Geometry check sheet. Reference: drawing and pictorial views, mm from the part's lowest x, y, z. A direction names the side the tool comes from. Round coordinates to 2 decimals unless told otherwise and drop trailing zeros. Write each loop counter-clockwise with the first axis right and the second up, starting at its lowest first coordinate (ties: lowest second). Pieces come first, ordered by that corner, then holes. Notation, with made-up numbers: (33.25, -37.75) - (63.25, -37.75) arc R8 ccw to (63.25, -31.75) - close; hole circle Ø1 at (65.25, -30). An arc over 180 degrees is marked (long way). Use one line per item in the form item = value. Start each with the question number.
1) Set-up check for the marked faces 4, 5 and 6: record each of +Z, -Z, +X, -X, +Y, -Y from which the full face is reachable in a straight line by a thin tool's end or side.
2) Section check B-B (y = 16). Record the boundary of the cut face in (x, z), then the cut area to 3 significant figures.
3) Section check C-C (x = 51). Record the boundary of the cut face in (y, z), then the cut area to 3 significant figures.
4) Gauge pin test, flat ends, axial feed: P1, Ø4, axis at x = 24, z = 19.5, coming from the +Y side; P2, Ø3, axis at y = 35, z = 13.5, coming from the +X side; P3, Ø12, axis at y = 13, z = 4, coming from the -X side; P4, Ø16, axis at y = 61, z = 14.5, coming from the +X side. Record the tip position at first contact, or that the pin passes through.
5) Draft check along X on the marked faces 1, 2 and 3. Enter one of: +X half, -X half, draft (parallel to the pull), parting line (faces both ways), or undercut.
6) Section check A-A (z = 7.75). Record the boundary of the cut face in (x, y).
7) Scan lines: probe 1 along Y at (x, z) = (48, 9.25); probe 2 along Z at (x, y) = (8.5, 44.5); probe 3 along Y at (x, z) = (6, 21.25). Record each from-to range of solid material in increasing order.
8) Section check D-D (x = 4). Record the boundary of the cut face in (y, z), then the cut area to 3 significant figures.
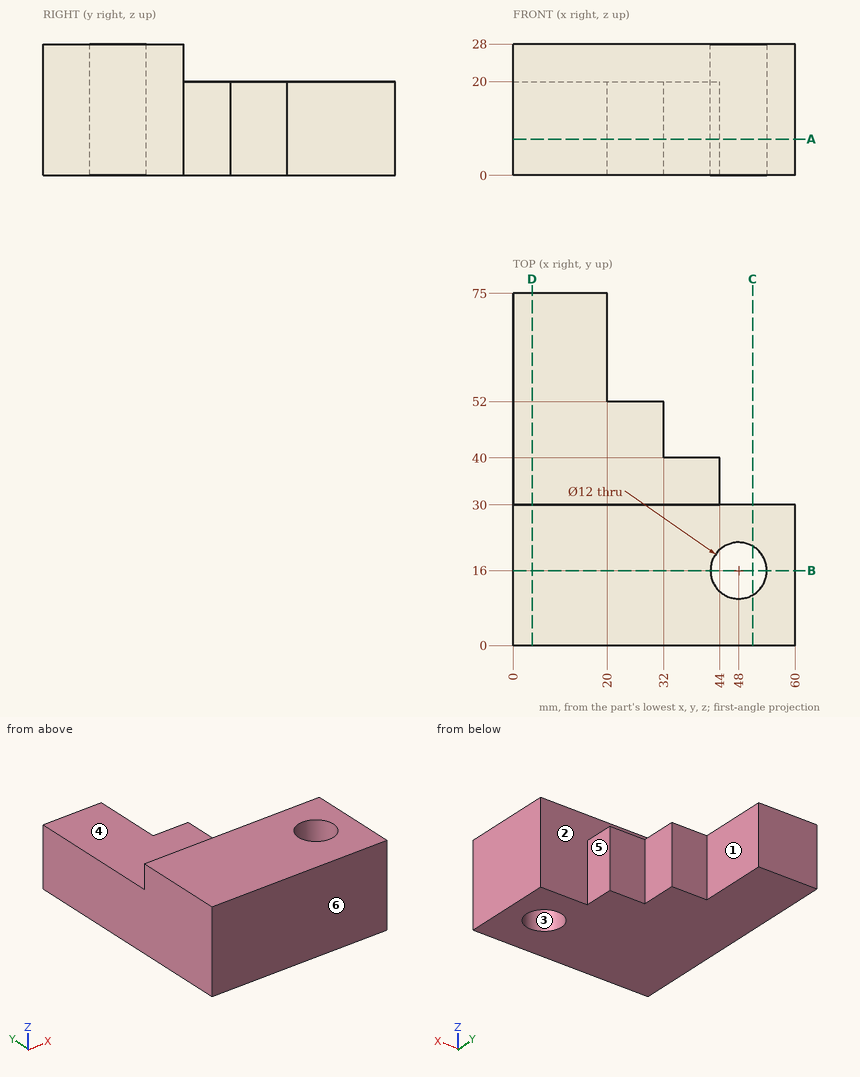
Results are:
q1.face_4 = +Z, +X, -X, +Y
q1.face_5 = +Z, -Z, +X, +Y
q1.face_6 = +Z, -Z, +X, -X, -Y
q2.outline = (0, 0) - (42, 0) - (42, 28) - (0, 28) - close; (54, 0) - (60, 0) - (60, 28) - (54, 28) - close
q2.area = 1,340 mm²
q3.outline = (0, 0) - (10.8, 0) - (10.8, 28) - (0, 28) - close; (21.2, 0) - (30, 0) - (30, 28) - (21.2, 28) - close
q3.area = 549 mm²
q4.P1 = 52
q4.P2 = 44
q4.P3 = 0
q4.P4 = 20
q5.face_1 = +X half
q5.face_2 = draft
q5.face_3 = undercut
q6.outline = (0, 0) - (60, 0) - (60, 30) - (44, 30) - (44, 40) - (32, 40) - (32, 52) - (20, 52) - (20, 75) - (0, 75) - close; hole circle Ø12 at (48, 16)
q7.probe_1 = 0 to 10, 22 to 30
q7.probe_2 = 0 to 20
q7.probe_3 = 0 to 30
q8.outline = (0, 0) - (75, 0) - (75, 20) - (30, 20) - (30, 28) - (0, 28) - close
q8.area = 1,740 mm²
